For this review, take the finished solid that the model builds, in its own axes (mm). Face numbers are marked on the shaded views. Round coordinates to 2 decimals unless told otherwise and drop trailing zeros. Order: outer loops, then holes, each group sorted by start corner. A loop starts at its lowest first (then second) coordinate and runs counter-clockwise, first axis right, second up. Notation, with made-up numbers: M 24,75 L 33,75 A30 cw 33,99 Z; hole C 35.25,69.5 d11. An arc over 180 degrees is marked long. Write item = value, one per line. Start each with the question number.
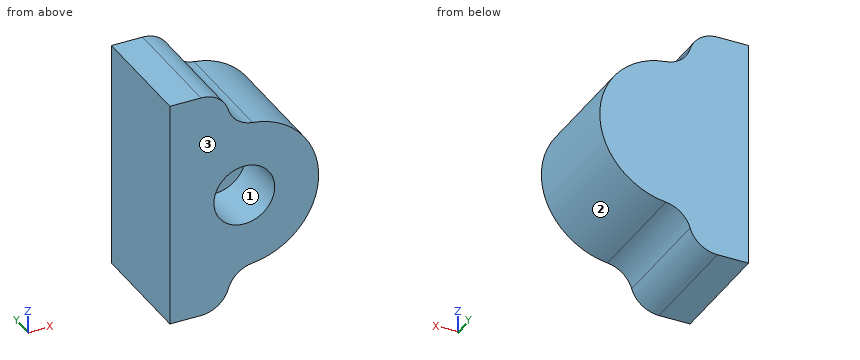
Autodesk Fusion 360 part; units mm, degrees
sketch "Sketch1" plane through (0, 0, 0) normal (0, 1, 0) x (1, 0, 0)
  circle A0 centre (0, 0) radius 3.175
  circle A1 centre (0, 0) radius 8.255
  line L0 (-1.905, -12.7) -> (-8.255, -12.7)
  line L1 (-8.255, -12.7) -> (-8.255, 12.7)
  line L2 (-8.255, 12.7) -> (-1.905, 12.7)
  line L3 (-1.905, 12.7) -> (-1.905, -12.7)
  circle A2 centre (1.27, -11.3592) radius 3.175
  circle A3 centre (1.27, 11.3592) radius 3.175
  circle A4 centre (0, 0) radius 3.375
  point P0 (-8.255, 0)
  dimension "d1" = 6.35
  dimension "d2" = 5.08
  dimension "d3" = 6.35
  dimension "d4" = 25.4
  dimension "d5" = 6.35
  dimension "d10" = 0.2
extrude "Extrude1" add sketch "Sketch1" along normal blind 12.7 contours A0 L3 | A0 L3 A4 | A0 L3 | A0 L3 A4 | A1 L3 A4 | A1 L3 A4 | A1 L3 A3 | A1 L1 L2 L3 | A1 L0 L1 L3 | A1 L3 A2
extrude "Extrude2" cut sketch "Sketch1" along normal blind 6.35 contours A0 L3 | A0 L3 A4 | A0 L3 | A0 L3 A4
fillet "Fillet5" radius 3.175 2 edges at (-1.905, 6.35, -12.7) (-1.905, 6.35, 12.7)
(1) For line 1 along Z through (x, y) = (1.5, 5.75); line 2 along Z through (x, y) = (0, 2.5) (3 decimals); line 3 along Y through (x, z) = (2, 0), list the stretches that pass through material, from the lowest coordinate up.
(2) We need section A-A, the plane z = 0. Write out the cut boundary in (x, y) (3 decimals), then the cut area to 3 significant figures.
(3) We need section D-D, the plane z = 10. Write out the cut boundary in (x, y) (3 decimals), then the cut area to 3 significant figures.
(4) We need section B-B, the plane x = 0. Write out the cut boundary in (y, z) (3 decimals).
(5) We need section C-C, the plane z = -6.5. Write out the cut boundary in (x, y) (3 decimals).
(6) Insertion check: pin 1 (5 mm diameter, centred on x = -4, z = -3, fed in from -Y); pin 2 (2 mm diameter, centred on x = -1.5, z = -1.5, fed in from -Y); pin 3 (4 mm diameter, centred on x = 2, y = 6, fed in from -Z). Each pin has a flat end and moves straight along its axis. Give the tip position at first contact, or say it passes through.
(7) Draft analysis for pull direction X (two halves, no side actions). For the marked faces 1, 2 and 3, state which applies: released by +X, released by -X, zero draft, split by the parting line, or undercut.
Values:
q1.line_1 = -8.12 to -3.02, 3.02 to 8.12
q1.line_2 = -8.449 to -3.375, 3.375 to 8.449
q1.line_3 = 6.35 to 12.7
q2.outline = M -8.255,0 L -3.375,0 L -3.375,6.35 L 3.375,6.35 L 3.375,0 L 8.255,0 L 8.255,12.7 L -8.255,12.7 Z
q2.area = 167 mm²
q3.outline = M -8.255,0 L -1.599,0 L -1.599,12.7 L -8.255,12.7 Z
q3.area = 84.5 mm²
q4.outline = M 0,-8.449 L 12.7,-8.449 L 12.7,8.449 L 0,8.449 L 0,3.375 L 6.35,3.375 L 6.35,-3.375 L 0,-3.375 Z
q5.outline = M -8.255,0 L 5.089,0 L 5.089,12.7 L -8.255,12.7 Z
q6.pin_1 = 0
q6.pin_2 = 6.35
q6.pin_3 = -8.45
q7.face_1 = undercut
q7.face_2 = released by +X
q7.face_3 = zero draft
